For this review, take the finished solid that the model builds, in its own axes (mm). Give positions to 0.01 mm unless a question says otherwise; leave off trailing zeros. Loops run counter-clockwise (first coordinate to the right, second up) from the corner with the lowest first, then second, coordinate; pieces in that order, holes last. Notation, with made-up numbers: (0, 78.25) - (16, 78.25) arc R18 cw to (16, 101.25) - close; hole circle Ø6 at (77.25, 68.25). An arc over 180 degrees is marked (long way). Answer in a Markdown table with one row per item.
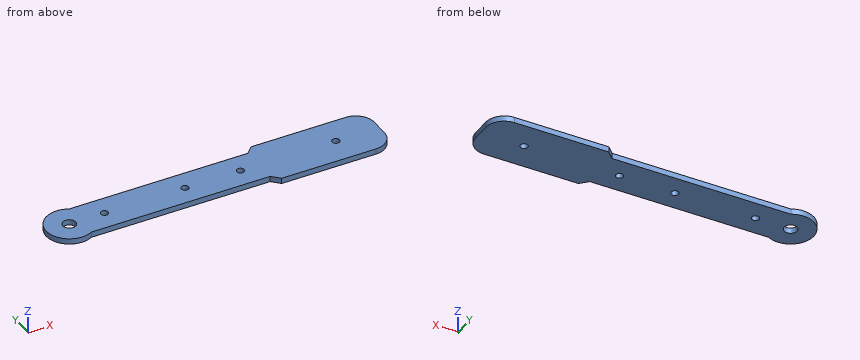
```python
from build123d import *

# Parameters (mm, degrees)
SALIENTE_EXTRUIR1_DEPTH = 3
REDONDEO1_R             = 10
CHAFL_N1_SIZE           = 4
CORTAR_EXTRUIR2_REACH   = 93.291
CROQUIS3_R              = 3.5
CROQUIS3_R_2            = 2
CORTAR_EXTRUIR3_REACH   = 93.291
CROQUIS4_R              = 2
CORTAR_EXTRUIR4_REACH   = 93.291
CROQUIS2_R              = 2


with BuildPart() as part:
    # Croquis1 → Saliente-Extruir1 (new body)
    with BuildSketch(Plane.XY):
        with BuildLine():
            Line((90, -15), (90, 15))
            Line((90, 15), (25, 15))
            Line((25, 15), (25, 11))
            Line((25, 11), (-25, 11))
            Line((-25, 11), (-71.562828956, 11))
            ThreePointArc((-71.562828956, 11), (-90, 0), (-71.562828956, -11))
            Line((-71.562828956, -11), (-25, -11))
            Line((-25, -11), (25, -11))
            Line((25, -11), (25, -15))
            Line((25, -15), (90, -15))
        make_face()
    extrude(amount=SALIENTE_EXTRUIR1_DEPTH)

    # Redondeo1
    redondeo1_edges = [part.edges().sort_by_distance(p)[0] for p in [
        (90, 15, 1.5),
        (90, -15, 1.5),
    ]]
    fillet(redondeo1_edges, radius=REDONDEO1_R)

    # Chaflán1
    chafl_n1_edges = [part.edges().sort_by_distance(p)[0] for p in [
        (25, -15, 1.5),
        (25, 15, 1.5),
    ]]
    chamfer(chafl_n1_edges, length=CHAFL_N1_SIZE - 0.0001)  # a hair under: the kernel refuses the full size

    # Croquis3 → Cortar-Extruir2 (cut, up to next)
    with BuildSketch(Plane.XY.offset(3), mode=Mode.PRIVATE) as cortar_extruir2_sk1:
        with Locations((-77.5, 0)):
            Circle(CROQUIS3_R)
    cortar_extruir2_tool1 = extrude(cortar_extruir2_sk1.sketch, amount=-CORTAR_EXTRUIR2_REACH, mode=Mode.PRIVATE) & part.part
    # Croquis3 → Cortar-Extruir2 (cut, up to next)
    with BuildSketch(Plane.XY.offset(3), mode=Mode.PRIVATE) as cortar_extruir2_sk2:
        with Locations((-58.5, 0)):
            Circle(CROQUIS3_R_2)
    cortar_extruir2_tool2 = extrude(cortar_extruir2_sk2.sketch, amount=-CORTAR_EXTRUIR2_REACH, mode=Mode.PRIVATE) & part.part
    add(cortar_extruir2_tool1.solids().sort_by_distance((-77.5, 0, 3))[0], mode=Mode.SUBTRACT)
    add(cortar_extruir2_tool2.solids().sort_by_distance((-58.5, 0, 3))[0], mode=Mode.SUBTRACT)

    # Croquis4 → Cortar-Extruir3 (cut, up to next)
    with BuildSketch(Plane.XY.offset(3), mode=Mode.PRIVATE) as cortar_extruir3_sk1:
        with Locations((-15, 0)):
            Circle(CROQUIS4_R)
    cortar_extruir3_tool1 = extrude(cortar_extruir3_sk1.sketch, amount=-CORTAR_EXTRUIR3_REACH, mode=Mode.PRIVATE) & part.part
    # Croquis4 → Cortar-Extruir3 (cut, up to next)
    with BuildSketch(Plane.XY.offset(3), mode=Mode.PRIVATE) as cortar_extruir3_sk2:
        with Locations((15, 0)):
            Circle(CROQUIS4_R)
    cortar_extruir3_tool2 = extrude(cortar_extruir3_sk2.sketch, amount=-CORTAR_EXTRUIR3_REACH, mode=Mode.PRIVATE) & part.part
    add(cortar_extruir3_tool1.solids().sort_by_distance((-15, 0, 3))[0], mode=Mode.SUBTRACT)
    add(cortar_extruir3_tool2.solids().sort_by_distance((15, 0, 3))[0], mode=Mode.SUBTRACT)

    # Croquis2 → Cortar-Extruir4 (cut, up to next)
    with BuildSketch(Plane.XY.offset(3), mode=Mode.PRIVATE) as cortar_extruir4_sk1:
        with Locations((66.5, 0)):
            Circle(CROQUIS2_R)
    cortar_extruir4_tool1 = extrude(cortar_extruir4_sk1.sketch, amount=-CORTAR_EXTRUIR4_REACH, mode=Mode.PRIVATE) & part.part
    add(cortar_extruir4_tool1.solids().sort_by_distance((66.5, 0, 3))[0], mode=Mode.SUBTRACT)


solid = part.part
```
1. We need section D-D, the plane x = -42.5. Give the boundary of the cut face in (y, z), and give its area (3 significant figures).
Values:
| item | result |
|---|---|
| outline | (-11, 0) - (11, 0) - (11, 3) - (-11, 3) - close |
| area | 66.0 mm^2 |
2. We need section B-B, the plane z = 0.75. Count the separate pieces of the cut face and the enclosed holes in it, and give its area (3 significant figures).
Values:
| item | result |
|---|---|
| separate pieces | 1 |
| enclosed holes | 5 |
| area | 4,310 mm^2 |
3. We need section A-A, the plane x = -15. Give the boundary of the cut face in (y, z), and give its area (3 significant figures).
Values:
| item | result |
|---|---|
| outline | (-11, 0) - (-2, 0) - (-2, 3) - (-11, 3) - close; (2, 0) - (11, 0) - (11, 3) - (2, 3) - close |
| area | 54.0 mm^2 |
4. We need section C-C, the plane y = 0. Give the boundary of the cut face in (x, z).
Values:
| item | result |
|---|---|
| outline | (-90, 0) - (-81, 0) - (-81, 3) - (-90, 3) - close; (-74, 0) - (-60.5, 0) - (-60.5, 3) - (-74, 3) - close; (-56.5, 0) - (-17, 0) - (-17, 3) - (-56.5, 3) - close; (-13, 0) - (13, 0) - (13, 3) - (-13, 3) - close; (17, 0) - (64.5, 0) - (64.5, 3) - (17, 3) - close; (68.5, 0) - (90, 0) - (90, 3) - (68.5, 3) - close |
5. Wall thickness on line 1 (Y direction, x = -15, z = 0.6); line 2 (Y direction, x = -77.5, z = 1.7); line 3 (X direction, y = -0.5, z = 1.15): over which ranges is each line inside the solid? List them lowest first. Write a range as [from, to].
Values:
| item | result |
|---|---|
| line 1 | y = [-11, -2], [2, 11] |
| line 2 | y = [-12.5, -3.5], [3.5, 12.5] |
| line 3 | x = [-89.99, -80.96], [-74.04, -60.44], [-56.56, -16.94], [-13.06, 13.06], [16.94, 64.56], [68.44, 90] |
6. Clearance check with flat-ended pins moving along their axes: pin 1 (1.5 mm diameter, centred on x = 3.5, z = 1.5, fed in from +Y); pin 2 (1.5 mm diameter, centred on y = 5.5, z = 2, fed in from -X). State where each tip first meets the part, or that it passes through.
Values:
| item | result |
|---|---|
| pin 1 | stops at y = 11 |
| pin 2 | stops at x = -89.06 |
